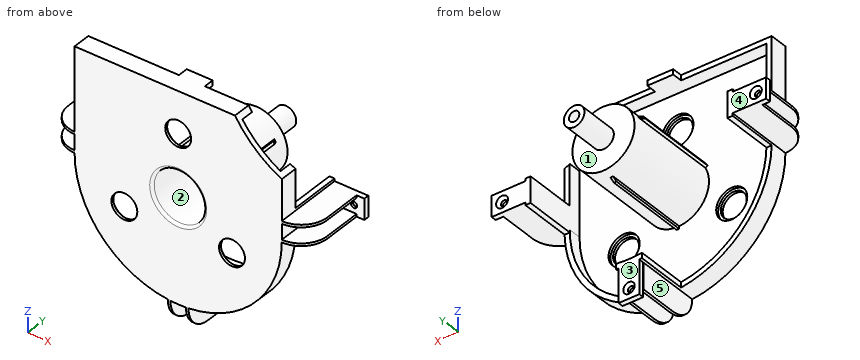
```python
from build123d import *

# Parameters (mm, degrees)
BOSS_EXTRUDE2_DEPTH                                 = 7
SHELL3_T                                            = -2
SKETCH2_R                                           = 12
BOSS_EXTRUDE3_DEPTH                                 = 40
SKETCH3_R                                           = 4
BOSS_EXTRUDE4_DEPTH                                 = 15
SHELL4_START                                        = 2
SHELL4_OUTLINE_R                                    = 10
SHELL4_DEPTH                                        = 36
SHELL4_START_2                                      = 38
SHELL4_2_OUTLINE_R                                  = 2
SHELL4_2_DEPTH                                      = 17
RIB1_START                                          = -0.5
RIB1_DEPTH                                          = 1
CIRPATTERN1_COUNT                                   = 3
BOSS_EXTRUDE5_DEPTH                                 = 2
SKETCH29_R                                          = 44.999999999999986
CUT_EXTRUDE14_DEPTH                                 = 7
BOSS_EXTRUDE9_DEPTH                                 = 2
SKETCH32_R                                          = 10
CUT_EXTRUDE10_DEPTH                                 = 2
FILLET3_R                                           = 1
SKETCH35_R                                          = 5.000000000000003
CUT_EXTRUDE12_DEPTH                                 = 2
CIRPATTERN2_COUNT                                   = 3
SKETCH37_R                                          = 6.000000000000001
CUT_EXTRUDE13_DEPTH                                 = 1
CIRPATTERN3_COUNT                                   = 3
BOSS_EXTRUDE13_DEPTH                                = 20
BOSS_EXTRUDE14_DEPTH                                = 2
BOSS_EXTRUDE15_DEPTH                                = 1
LPATTERN4_COUNT                                     = 2
LPATTERN4_PITCH                                     = 7
FILLET4_R                                           = 10
CSK_FOR_M2_COUNTERSUNK_FLAT_HEAD_SCREW6_D           = 2.4
CSK_FOR_M2_COUNTERSUNK_FLAT_HEAD_SCREW6_CSINK_D     = 4.4
CSK_FOR_M2_COUNTERSUNK_FLAT_HEAD_SCREW6_CSINK_ANGLE = 90
BOSS_EXTRUDE16_DEPTH                                = 2
SKETCH68_W                                          = 10
SKETCH68_H                                          = 25.000000000000004
EXTRUDE_THIN1_DEPTH                                 = 1
LPATTERN5_COUNT                                     = 2
LPATTERN5_PITCH                                     = 7
LPATTERN6_COUNT                                     = 2
LPATTERN6_PITCH                                     = 78
LPATTERN7_COUNT                                     = 2
LPATTERN7_PITCH                                     = 93
LPATTERN8_COUNT                                     = 2
LPATTERN8_PITCH                                     = 90
LPATTERN8_COPY_1_SKETCH_W                           = 10
LPATTERN8_COPY_1_SKETCH_H                           = 25.000000000000004
LPATTERN8_COPY_1_DEPTH                              = 1
FILLET5_R                                           = 10
CSK_FOR_M2_FLAT_CROSS_HEAD_SCREW1_D                 = 2.4
CSK_FOR_M2_FLAT_CROSS_HEAD_SCREW1_CSINK_D           = 4.6
CSK_FOR_M2_FLAT_CROSS_HEAD_SCREW1_CSINK_ANGLE       = 92


# Read off the part's stored shape, not the designer's step: Shell4, Rib1
with BuildPart() as part:
    # Sketch1 → Boss-Extrude2 (new body)
    with BuildSketch(Plane(origin=(0, 0, 0), x_dir=(1, 0, 0), z_dir=(0, 1, 0))):
        with BuildLine():
            Line((40, 4.9e-15), (40.00000000000001, -40.00000000000001))
            Line((40.00000000000001, -40.00000000000001), (-40.00000000000001, -40.00000000000001))
            Line((-40.00000000000001, -40.00000000000001), (-40, 4.9e-15))
            ThreePointArc((-40, 4.9e-15), (-6.43e-15, 40), (40, 4.9e-15))
        make_face()
    extrude(amount=BOSS_EXTRUDE2_DEPTH)

    # Shell3
    shell3_openings = [part.faces().sort_by_distance(p)[0] for p in [
        (0, 7, 3.733994357),
    ]]
    offset(amount=SHELL3_T, openings=shell3_openings, kind=Kind.INTERSECTION)

    # Sketch2 → Boss-Extrude3 (add)
    with BuildSketch(Plane(origin=(0, 0, 0), x_dir=(1, 0, 0), z_dir=(0, 1, 0))):
        with Locations(Location((0, 0, 0), (0, 0, 270))):
            Circle(SKETCH2_R)
    extrude(amount=BOSS_EXTRUDE3_DEPTH)

    # Sketch3 → Boss-Extrude4 (add)
    with BuildSketch(Plane(origin=(0, 40, 0), x_dir=(1, 0, 0), z_dir=(0, 1, 0))):
        with Locations(Location((0, 0, 0), (0, 0, 270))):
            Circle(SKETCH3_R)
    extrude(amount=BOSS_EXTRUDE4_DEPTH)

    # Shell4 outline → Shell4 (cut)
    with BuildSketch(Plane(origin=(0, 0, 0), x_dir=(1, 0, 0), z_dir=(0, 1, 0)).offset(SHELL4_START)):
        Circle(SHELL4_OUTLINE_R)
    extrude(amount=SHELL4_DEPTH, mode=Mode.SUBTRACT)

    # Shell4 2 outline → Shell4 2 (cut)
    with BuildSketch(Plane(origin=(0, 0, 0), x_dir=(1, 0, 0), z_dir=(0, 1, 0)).offset(SHELL4_START_2)):
        Circle(SHELL4_2_OUTLINE_R)
    extrude(amount=SHELL4_2_DEPTH, mode=Mode.SUBTRACT)

    # Rib1 outline → Rib1 (add)
    with BuildSketch(Plane(origin=(0, 0, 0), x_dir=(0, 0, -1), z_dir=(1, 0, 0)).offset(RIB1_START)):
        Polygon((13, 34), (11.989578808, 35.750100841), (11.267949192, 37), (10, 37), (10, 1), (13, 1), align=None)
    rib1 = extrude(amount=RIB1_DEPTH)

    # CirPattern1: Rib1 ×3 about axis
    cirpattern1_axis = Axis((-5e-17, 0, 1.3e-15), (0, 1, 0))
    for i in range(1, CIRPATTERN1_COUNT):
        add(rib1.rotate(cirpattern1_axis, i * 360 / CIRPATTERN1_COUNT))

    # Sketch13 → Boss-Extrude5 (add)
    with BuildSketch(Plane(origin=(40, 0, -6.94e-15), x_dir=(0, 0, -1), z_dir=(1, 0, 0))):
        Polygon((0.9999999999999784, 7.0000000000000036), (0.9999999999999662, 27.000000000000004), (-9.000000000000014, 27), (-9.000000000000014, 7), (-40.000000000000014, 7), (-40.000000000000014, 0), (0, 0), (0, 7), align=None)
    boss_extrude5 = extrude(amount=-BOSS_EXTRUDE5_DEPTH)

    # Sketch29 → Cut-Extrude14 (cut)
    with BuildSketch(Plane(origin=(0, 0, 0), x_dir=(1, 0, 0), z_dir=(0, 1, 0))):
        with Locations((60.00000000000001, -64)):
            Circle(SKETCH29_R)
    extrude(amount=CUT_EXTRUDE14_DEPTH, mode=Mode.SUBTRACT)

    # Sketch31 → Boss-Extrude9 (add)
    with BuildSketch(Plane.XY.offset(40.00000000000001)):
        Polygon((5, 0), (5, 11), (-5.0000000000000036, 11), (-5, 0), align=None)
    extrude(amount=-BOSS_EXTRUDE9_DEPTH)

    # Sketch32 → Cut-Extrude10 (cut)
    with BuildSketch(Plane(origin=(0, 0, 0), x_dir=(1, 0, 0), z_dir=(0, 1, 0))):
        with Locations(Location((0, 0, 0), (0, 0, 270))):
            Circle(SKETCH32_R)
    extrude(amount=CUT_EXTRUDE10_DEPTH, mode=Mode.SUBTRACT)

    # Fillet3
    fillet3_edges = [part.edges().sort_by_distance(p)[0] for p in [
        (3.06e-15, 0, -10),
    ]]
    fillet(fillet3_edges, radius=FILLET3_R)

    # Sketch35 → Cut-Extrude12 (cut)
    with BuildSketch(Plane(origin=(0, 2, 0), x_dir=(1, 0, 0), z_dir=(0, 1, 0))):
        with Locations(Location((0, -24, 0), (0, 0, 270))):
            Circle(SKETCH35_R)
    cut_extrude12 = extrude(amount=-CUT_EXTRUDE12_DEPTH, mode=Mode.SUBTRACT)

    # CirPattern2: Cut-Extrude12 ×3 about axis
    cirpattern2_axis = Axis((-3.7e-16, 0, -1.37e-15), (0, 1, 0))
    for i in range(1, CIRPATTERN2_COUNT):
        add(cut_extrude12.rotate(cirpattern2_axis, i * 360 / CIRPATTERN2_COUNT), mode=Mode.SUBTRACT)

    # Sketch37 → Cut-Extrude13 (cut)
    with BuildSketch(Plane(origin=(0, 2, 0), x_dir=(1, 0, 0), z_dir=(0, 1, 0))):
        with Locations(Location((0, -24, 0), (0, 0, 270))):
            Circle(SKETCH37_R)
    cut_extrude13 = extrude(amount=-CUT_EXTRUDE13_DEPTH, mode=Mode.SUBTRACT)

    # CirPattern3: Cut-Extrude13 ×3 about axis
    cirpattern3_axis = Axis((3.7e-16, 0, -1.37e-15), (0, 1, 0))
    for i in range(1, CIRPATTERN3_COUNT):
        add(cut_extrude13.rotate(cirpattern3_axis, i * 360 / CIRPATTERN3_COUNT), mode=Mode.SUBTRACT)

    # Sketch61 → Boss-Extrude13 (add)
    with BuildSketch(Plane(origin=(0, 7, 0), x_dir=(1, 0, 0), z_dir=(0, 1, 0))):
        with BuildLine():
            Line((5, 39.68626966596886), (5.000000000000001, 37.66961640367472))
            ThreePointArc((5.000000000000001, 37.66961640367472), (2.33e-15, 38), (-5, 37.66961640367472))
            Line((-5, 37.66961640367472), (-5, 39.68626966596886))
            ThreePointArc((-5, 39.68626966596886), (2.45e-15, 40), (5, 39.68626966596886))
        make_face()
    extrude(amount=BOSS_EXTRUDE13_DEPTH)



with BuildPart() as body_2:
    # Sketch62 → Boss-Extrude14 (new body)
    with BuildSketch(Plane(origin=(0, 27, 0), x_dir=(1, 0, 0), z_dir=(0, 1, 0))):
        with BuildLine():
            Line((-3.9891832676658594, 52.80058312207215), (-3.9891832676658594, 39.800583122072155))
            ThreePointArc((-3.9891832676658567, 39.800583122072155), (2.45e-15, 40), (3.9891832676658616, 39.800583122072155))
            Line((3.9891832676658594, 39.800583122072155), (3.9891832676658594, 52.80058312207215))
            Line((3.9891832676658594, 52.80058312207215), (-3.9891832676658594, 52.80058312207215))
        make_face()
    extrude(amount=-BOSS_EXTRUDE14_DEPTH)


with BuildPart() as part_1:
    add(part.part)

    add(body_2.part)  # Boss-Extrude15 merges body 2
    # Sketch63 → Boss-Extrude15 (add)
    with BuildSketch(Plane(origin=(3.9891832676658594, 0, 0), x_dir=(0, 0, -1), z_dir=(1, 0, 0))):
        Polygon((49.800583122072155, 25), (49.800583122072155, 9.75e-15), (40, 0), (39.80058312207216, 0), (39.80058312207216, 25), align=None)
    boss_extrude15 = extrude(amount=-BOSS_EXTRUDE15_DEPTH)

    # LPattern4: Boss-Extrude15 ×2
    with Locations(*[(-i * LPATTERN4_PITCH, 0, 0) for i in range(1, LPATTERN4_COUNT)]):
        add(boss_extrude15)

    # Fillet4
    fillet4_edges = [part_1.edges().sort_by_distance(p)[0] for p in [
        (-3.5108167323341406, 9.75e-15, -49.800583122072155),
    ]]
    fillet(fillet4_edges, radius=FILLET4_R)

    # CSK for M2 Countersunk Flat Head Screw6 (through all)
    with Locations(Plane(origin=(0, 27, 0), x_dir=(1, 0, 0), z_dir=(0, 1, 0))):
        with Locations((0, 48.800583122)):
            CounterSinkHole(CSK_FOR_M2_COUNTERSUNK_FLAT_HEAD_SCREW6_D / 2, CSK_FOR_M2_COUNTERSUNK_FLAT_HEAD_SCREW6_CSINK_D / 2, counter_sink_angle=CSK_FOR_M2_COUNTERSUNK_FLAT_HEAD_SCREW6_CSINK_ANGLE)

    # Sketch67 → Boss-Extrude16 (add)
    with BuildSketch(Plane(origin=(0, 27.000000000000004, 9.37e-15), x_dir=(1, 0, 0), z_dir=(0, 1, 3.5e-16))):
        Polygon((40, -8.67e-15), (53, -8.67e-15), (53, -4.000000000000009), (53, -8.000000000000009), (40, -8.000000000000009), align=None)
    boss_extrude16 = extrude(amount=-BOSS_EXTRUDE16_DEPTH)

    # Sketch68 → Extrude-Thin1 (add)
    with BuildSketch(Plane.XY.offset(8.000000000000009)):
        with Locations((45.00000000000001, 12.500000000000002)):
            Rectangle(SKETCH68_W, SKETCH68_H)
    extrude_thin1 = extrude(amount=-EXTRUDE_THIN1_DEPTH)

    # LPattern5: Extrude-Thin1 ×2
    with Locations(*[(0, 0, -i * LPATTERN5_PITCH) for i in range(1, LPATTERN5_COUNT)]):
        add(extrude_thin1)

    # LPattern6: Boss-Extrude5 ×2
    with Locations(*[(-i * LPATTERN6_PITCH, 0, 0) for i in range(1, LPATTERN6_COUNT)]):
        add(boss_extrude5)

    # LPattern7: Boss-Extrude16 ×2
    with Locations(*[(-i * LPATTERN7_PITCH, 0, 0) for i in range(1, LPATTERN7_COUNT)]):
        add(boss_extrude16)

    # LPattern8: Extrude-Thin1 ×2
    with Locations(*[(-i * LPATTERN8_PITCH, 0, 0) for i in range(1, LPATTERN8_COUNT)]):
        add(extrude_thin1)

    # LPattern8 copy 1 sketch → LPattern8 copy 1 (add)
    with BuildSketch(Plane(origin=(-90, -2.78e-15, 0.9999999999999929), x_dir=(1, 0, 0), z_dir=(0, 0, 1))):
        with Locations((45.00000000000001, 12.500000000000002)):
            Rectangle(LPATTERN8_COPY_1_SKETCH_W, LPATTERN8_COPY_1_SKETCH_H)
    extrude(amount=-LPATTERN8_COPY_1_DEPTH)

    # Fillet5
    fillet5_edges = [part_1.edges().sort_by_distance(p)[0] for p in [
        (-49.99999999999999, -2.8e-15, 7.499999999999993),
        (-49.99999999999999, -2.8e-15, 0.4999999999999929),
        (50.00000000000001, -2.8e-15, 7.500000000000009),
        (50.00000000000001, -2.8e-15, 0.5000000000000089),
    ]]
    fillet(fillet5_edges, radius=FILLET5_R)

    # CSK for M2 Flat Cross Head Screw1 (through all)
    with Locations(Plane(origin=(0, 27.000000000000004, 9.37e-15), x_dir=(1, 0, 0), z_dir=(0, 1, 3.5e-16))):
        with Locations((49, -4), (-49, -4)):
            CounterSinkHole(CSK_FOR_M2_FLAT_CROSS_HEAD_SCREW1_D / 2, CSK_FOR_M2_FLAT_CROSS_HEAD_SCREW1_CSINK_D / 2, counter_sink_angle=CSK_FOR_M2_FLAT_CROSS_HEAD_SCREW1_CSINK_ANGLE)


solid = part_1.part
```
For this review, take the finished solid that the model builds, in its own axes (mm). Face numbers are marked on the shaded views. A direction names the side the tool comes from. Coordinates: 2 decimals unless noted, no trailing zeros. Order: outer loops, then holes, each group sorted by start corner. A loop starts at its lowest first (then second) coordinate and runs counter-clockwise, first axis right, second up. Notation, with made-up numbers: (83.25, 4) - (90.25, 4) arc R28 cw to (90.25, 32) - close; hole circle Ø3 at (-37.75, -31). An arc over 180 degrees is marked (long way). Answer as a JSON object with one key per item and string values. Group by question number.
1. We need section A-A on y = 28.5. State the section outline as (x, z) points, then the cut area to 3 significant figures.
2. We need section B-B on z = -23. State the section outline as (x, y) points, then the cut area to 3 significant figures.
3. For probe 1 along X at (y, z) = (8.5, -45); probe 2 along X at (y, z) = (47.75, 0); probe 3 along Z at (x, y) = (-47, 13), list the stretches that pass through material, from the lowest coordinate up.
4. For the marked faces 1, 2, 3, 4 and 5, list the 3-axis set-ups (+Z, -Z, +X, -X, +Y, -Y) from which the entire face can be reached by the end or side of a thin tool; tool diameter is ignored.
5. We need section C-C on y = 18.5. Give the number of separate pieces and of enclosed holes in the cut face, then the cut area to 3 significant figures.
6. Clearance check with flat-ended pins moving along their axes: P1, Ø0.5, axis at y = 20.5, z = 7.5, coming from the +X side; P2, Ø8, axis at x = 8, y = 42.5, coming from the +Z side; P3, Ø5, axis at x = -23.5, z = -21, coming from the +Y side. State where each tip first meets the part, or that it passes through.
7. We need section D-D on y = 49. State the section outline as (x, z) points.
Final values:
{
 "1": {"outline": "(-11.51, 6.07) - (-10.63, 5.56) arc R12 ccw to (-0.5, -11.99) - (-0.5, -13) - (0.5, -13) - (0.5, -11.99) arc R12 ccw to (10.63, 5.56) - (11.51, 6.07) - (11.01, 6.93) - (10.13, 6.43) arc R12 ccw to (-10.13, 6.43) - (-11.01, 6.93) - close; hole circle Ø20 at (0, 0)", "area": "141 mm²"},
 "2": {"outline": "(-32.73, 0) - (32.73, 0) - (32.73, 7) - (30.25, 7) - (30.25, 2) - (-30.25, 2) - (-30.25, 7) - (-32.73, 7) - close", "area": "156 mm²"},
 "3": {"probe 1": "-4.01 to -3.01, 2.99 to 3.99", "probe 2": "-4 to -2, 2 to 4", "probe 3": "0 to 1, 7 to 8"},
 "4": {"face 1": "+Y", "face 2": "-Y", "face 3": "-Z, +X, -X, +Y", "face 4": "+Z, -Z, -X, +Y", "face 5": "-Z, -X, +Y, -Y"},
 "5": {"separate pieces": "4", "enclosed holes": "1", "area": "261 mm²"},
 "6": {"P1": "x = 50", "P2": "z = 10.96", "P3": "y = 2"},
 "7": {"outline": "circle Ø8 at (0, 0); hole circle Ø4 at (0, 0)"}
}
